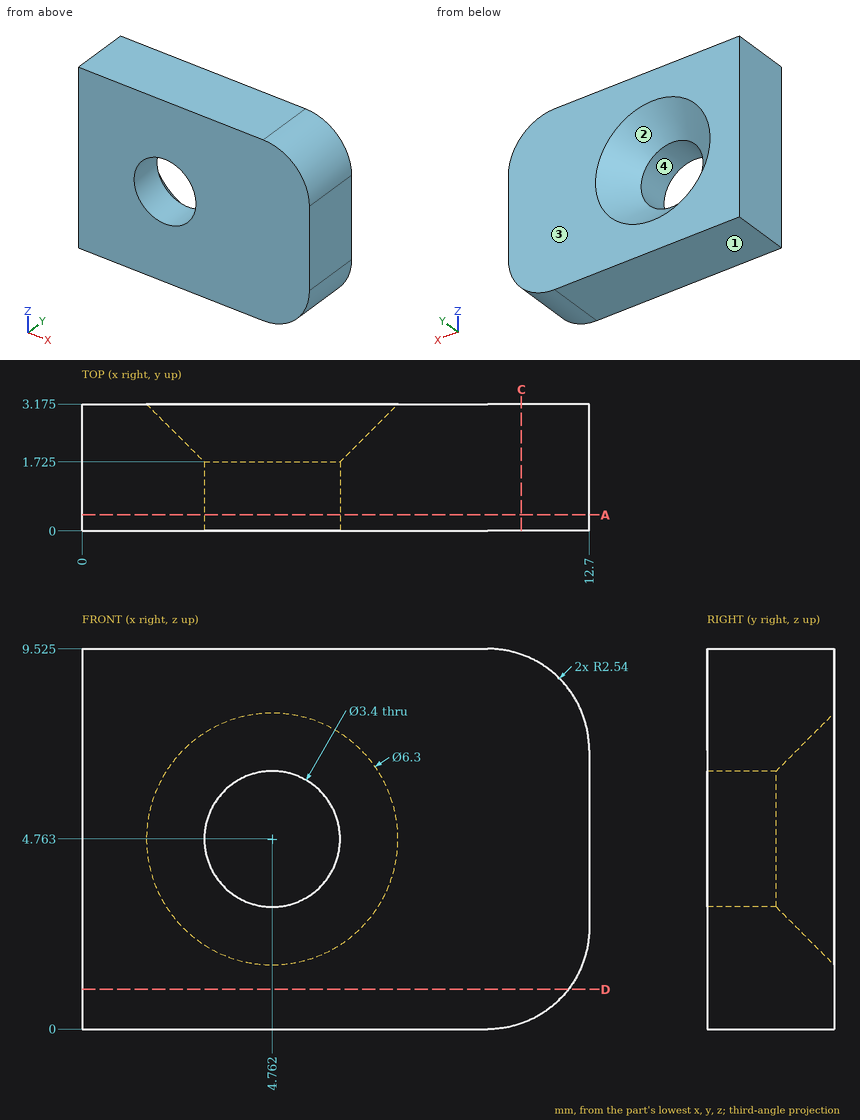
Geometry: see drawing. Coordinates: mm, zero at the bounding-box minimum. Coordinates: 2 decimals unless noted, no trailing zeros. Loops run counter-clockwise (first coordinate to the right, second up) from the corner with the lowest first, then second, coordinate; pieces in that order, holes last. Notation, with made-up numbers: M 45,86 L 90,86 A28 ccw 90,120 Z; hole C 62,64.25 d10. An arc over 180 degrees is marked long. Answer in a Markdown table with one row per item.
Q1. Section D-D on z = 1. Return the cut outline in (x, y) (1 decimal).
Answers below:
| item | result |
|---|---|
| outline | M 0,0 L 12.2,0 L 12.2,3.2 L 0,3.2 Z |
Q2. First-contact query: pin 1 (2 mm diameter, centred on x = 4.76, z = 4.76, fed in from -Y). Flat tip, straight axial feed; report the tip coordinate or a pass-through.
Answers below:
| item | result |
|---|---|
| pin 1 | passes through |
Q3. Section C-C on x = 11. Return the cut outline in (y, z) (1 decimal).
Answers below:
| item | result |
|---|---|
| outline | M 0,0.1 L 3.2,0.1 L 3.2,9.4 L 0,9.4 Z |
Q4. Ray query, probe 1 along X at (y, z) = (2.2, 5) (1 decimal); probe 2 along Z at (x, y) = (4, 0.9) (1 decimal); probe 3 along Z at (x, y) = (6, 1.7) (1 decimal). Return the intervals inside material, ascending. Write a range as from..to.
Answers below:
| item | result |
|---|---|
| probe 1 | x = 0..2.6, 6.9..12.7 |
| probe 2 | z = 0..3.2, 6.3..9.5 |
| probe 3 | z = 0..3.6, 5.9..9.5 |
Q5. Draft query along Z for the marked faces 1, 2, 3 and 4. Return one class per face: pulls with the +Z half, pulls with the -Z half, needs draft (parallel to the pull), parting line crosses it, or undercut.
Answers below:
| item | result |
|---|---|
| face 1 | pulls with the -Z half |
| face 2 | undercut |
| face 3 | needs draft |
| face 4 | undercut |
Q6. Section A-A on y = 0.4. Return the cut outline in (x, z) (1 decimal).
Answers below:
| item | result |
|---|---|
| outline | M 0,0 L 10.2,0 A2.5 ccw 12.7,2.5 L 12.7,7 A2.5 ccw 10.2,9.5 L 0,9.5 Z; hole C 4.8,4.8 d3.4 |
